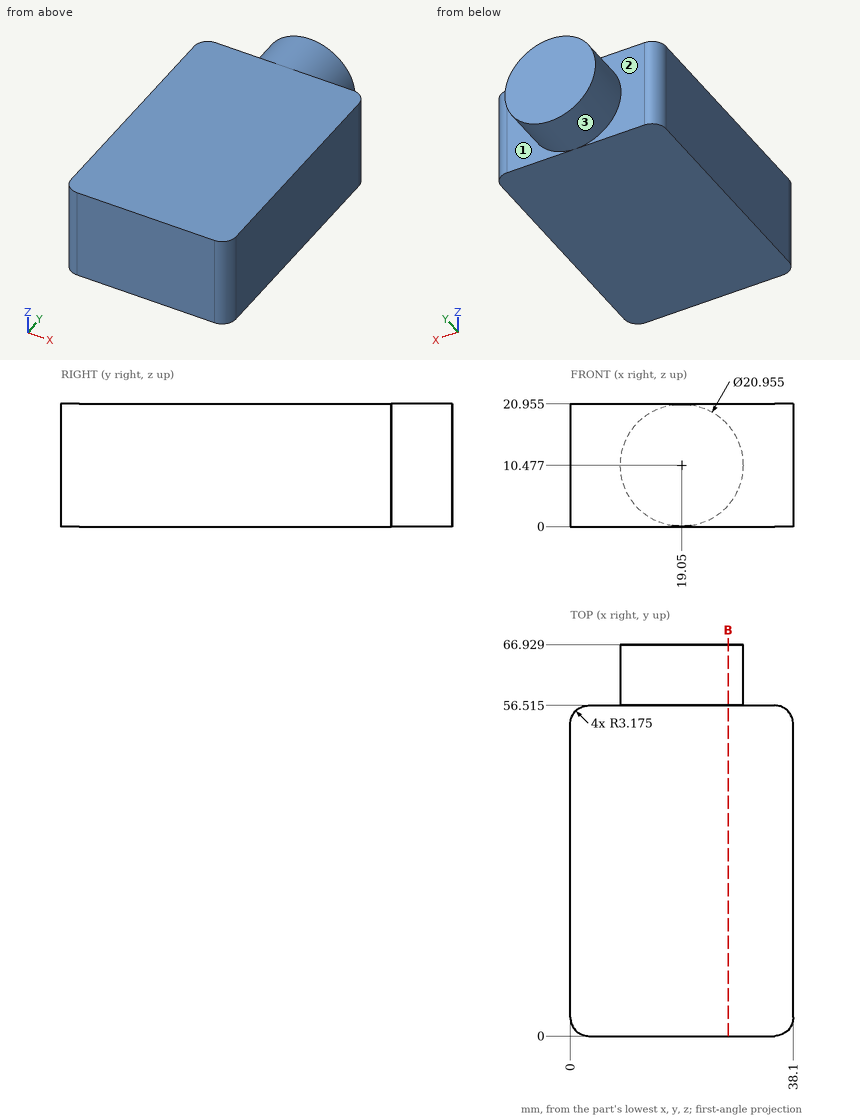
Here's the drawing with two shaded views (mm, measured from the low corner). I have some questions. A direction names the side the tool comes from. Coordinates: 2 decimals unless noted, no trailing zeros. Write each loop counter-clockwise with the first axis right and the second up, starting at its lowest first coordinate (ties: lowest second). Pieces come first, ordered by that corner, then holes. Notation, with made-up numbers: (-40, -26.5) -> (-26, -26.5) arc R23 ccw to (-26, 3.5) -> close; hole circle Ø11 at (13, 17.25). An arc over 180 degrees is marked (long way). Write item = value, one per line. Start each with the question number.
(1) Which directions (+Z, -Z, +X, -X, +Y, -Y) give clear straight access to the entire face, cutting with the end or side of a thin tool? Please do the marked faces 1, 2 and 3.
(2) Will this pin go through, and if not, where does the flat tip stop? pin 1 (1 mm diameter, centred on x = 31, z = 18, fed in from +Y) (1 decimal).
(3) I need wall thicknesses on line 1 (Y direction, x = 8.5, z = 1) (1 decimal); line 2 (X direction, y = 64.5, z = 2) (1 decimal); line 3 (Z direction, x = 21, y = 62). Which ranges of each line are inside material? Lowest first, please. Write a range as [from, to].
(4) I want a section at B-B (x = 27). Please give me the cut outline in (y, z) (1 decimal).
Result set:
q1.face_1 = +X, +Y
q1.face_2 = -X, +Y
q1.face_3 = +Y
q2.pin_1 = 56.5
q3.line_1 = [0, 56.5]
q3.line_2 = [12.9, 25.2]
q3.line_3 = [0.18, 20.77]
q4.outline = (0, 0) -> (56.5, 0) -> (56.5, 3.7) -> (66.9, 3.7) -> (66.9, 17.3) -> (56.5, 17.3) -> (56.5, 21) -> (0, 21) -> close
